Job drawing, mm, ordinate dimensions from the low corner. One solid piece. A direction names the side the tool comes from. Give positions to 0.01 mm unless a question says otherwise; leave off trailing zeros. Write each loop counter-clockwise with the first axis right and the second up, starting at its lowest first coordinate (ties: lowest second). Pieces come first, ordered by that corner, then holes. Notation, with made-up numbers: (23.5, 46) - (77.5, 46) arc R29 cw to (77.5, 81) - close; hole circle Ø8 at (34.25, 25). An arc over 180 degrees is marked (long way). Use a Markdown table: item, result. Add a question column.
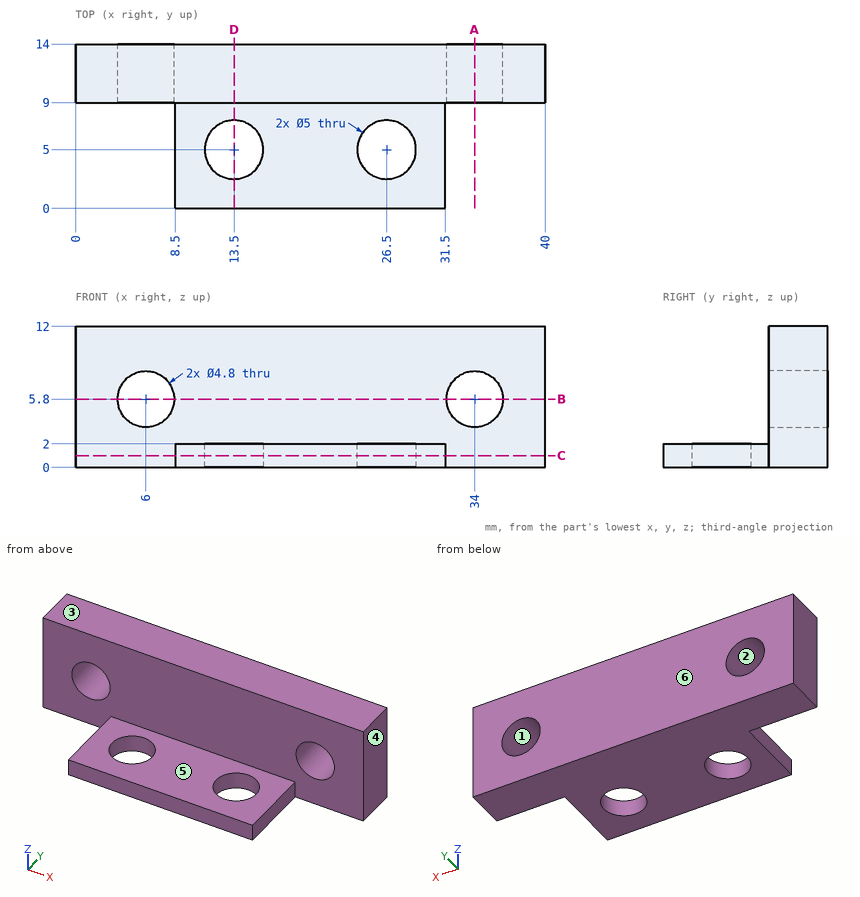
(1) Which spindle directions (+Z, -Z, +X, -X, +Y, -Y) get a long thin tool onto all of the face, cutting with end or side? Do the marked faces 5 and 6. Say none if no direction does.
(2) Band-saw the part on A-A (x = 34). Write the cut outline in (y, z).
(3) Two-plate mould, pull along Z, no slides. Class the marked faces 1, 2, 3 and 4: +Z half, -Z half, draft (parallel to the pull), parting line (faces both ways), or undercut.
(4) Band-saw the part on B-B (z = 5.8). Write the cut outline in (x, y), then the cut area to 3 significant figures.
(5) Band-saw the part on D-D (x = 13.5). Write the cut outline in (y, z), then the cut area to 3 significant figures.
(6) Band-saw the part on C-C (z = 1). Write the cut outline in (x, y).
(7) Flat gauge pins, fed straight in: pin 1 (1 mm diameter, centred on y = 3.5, z = 0.5, fed in from +X); pin 2 (2.5 mm diameter, centred on x = 16.5, y = 6, fed in from +Z); pin 3 (1 mm diameter, centred on y = 4, z = 1, fed in from -X). Where does each tip first touch, or does it go through?
(8) Probe probe 1 along X at (y, z) = (10.1, 5.8); probe 2 along X at (y, z) = (11, 3.75); probe 3 along Y at (x, z) = (26.5, 1.45). List the from-to ranges inside material, lowest first. Write a range as [from, to].
Model answer:
| question | item | result |
|---|---|---|
| 1 | face 5 | +Z, +X, -X, -Y |
| 1 | face 6 | +Z, -Z, +X, -X, +Y |
| 2 | outline | (9, 0) - (14, 0) - (14, 3.4) - (9, 3.4) - close; (9, 8.2) - (14, 8.2) - (14, 12) - (9, 12) - close |
| 3 | face 1 | undercut |
| 3 | face 2 | undercut |
| 3 | face 3 | +Z half |
| 3 | face 4 | draft |
| 4 | outline | (0, 9) - (3.6, 9) - (3.6, 14) - (0, 14) - close; (8.4, 9) - (31.6, 9) - (31.6, 14) - (8.4, 14) - close; (36.4, 9) - (40, 9) - (40, 14) - (36.4, 14) - close |
| 4 | area | 152 mm^2 |
| 5 | outline | (0, 0) - (2.5, 0) - (2.5, 2) - (0, 2) - close; (7.5, 0) - (14, 0) - (14, 12) - (9, 12) - (9, 2) - (7.5, 2) - close |
| 5 | area | 68.0 mm^2 |
| 6 | outline | (0, 9) - (8.5, 9) - (8.5, 0) - (31.5, 0) - (31.5, 9) - (40, 9) - (40, 14) - (0, 14) - close; hole circle Ø5 at (13.5, 5); hole circle Ø5 at (26.5, 5) |
| 7 | pin 1 | stops at x = 31.5 |
| 7 | pin 2 | stops at z = 2 |
| 7 | pin 3 | stops at x = 8.5 |
| 8 | probe 1 | x = [0, 3.6], [8.4, 31.6], [36.4, 40] |
| 8 | probe 2 | x = [0, 4.75], [7.25, 32.75], [35.25, 40] |
| 8 | probe 3 | y = [0, 2.5], [7.5, 14] |
